Autodesk Inventor part; units mm, degrees
ref_plane "YZ Plane" through (0, 0, 0) normal (1, 0, 0) x (0, 1, 0)
ref_plane "XZ Plane" through (0, 0, 0) normal (0, 1, 0) x (-1, 0, 0)
ref_plane "XY Plane" through (0, 0, 0) normal (0, 0, 1) x (1, 0, 0)
sketch "Sketch1" plane through (0, 0, 0) normal (0, 0, 1) x (1, 0, 0)
  line L0 (-14.5, 25.1147) -> (14.5, 25.1147) construction
  line L1 (14.5, 25.1147) -> (29, 0) construction
  line L2 (29, 0) -> (14.5, -25.1147) construction
  line L3 (14.5, -25.1147) -> (-14.5, -25.1147) construction
  line L4 (-14.5, -25.1147) -> (-29, 0) construction
  line L5 (-29, 0) -> (-14.5, 25.1147) construction
  line L6 (-18.7639, 32.5) -> (18.7639, 32.5)
  line L7 (18.7639, 32.5) -> (37.5278, 0)
  line L8 (37.5278, 0) -> (18.7639, -32.5)
  line L9 (18.7639, -32.5) -> (-18.7639, -32.5)
  line L10 (-18.7639, -32.5) -> (-37.5278, 0)
  line L11 (-37.5278, 0) -> (-18.7639, 32.5)
  circle A0 centre (-14.5, 25.1147) radius 11 construction
  circle A1 centre (14.5, 25.1147) radius 11 construction
  circle A2 centre (29, 0) radius 11 construction
  circle A3 centre (14.5, -25.1147) radius 11 construction
  circle A4 centre (-14.5, -25.1147) radius 11 construction
  circle A5 centre (-29, 0) radius 11 construction
  circle A6 centre (-14.5, 25.1147) radius 4
  circle A7 centre (14.5, 25.1147) radius 4
  circle A8 centre (29, 0) radius 4
  circle A9 centre (14.5, -25.1147) radius 4
  circle A10 centre (-14.5, -25.1147) radius 4
  circle A11 centre (-29, 0) radius 4
  circle A12 centre (0, 0) radius 4
  circle A13 centre (0, 0) radius 40 construction
  circle A14 centre (0, 0) radius 37.5278 construction
  dimension "d17" = 75.0555
  dimension "d0" = 22
  dimension "d1" = 50.2295
  dimension "d2" = 8
  dimension "d3" = 65
  dimension "d4" = 8
  dimension "d13" = 80
extrude "Extrusion1" add sketch "Sketch1" along normal blind 5
fillet "Fillet1" radius 4 6 edges at (37.5278, 0, 2.5) (18.7639, -32.5, 2.5) (-18.7639, -32.5, 2.5) (-37.5278, 0, 2.5) (-18.7639, 32.5, 2.5) (18.7639, 32.5, 2.5)
sketch "Sketch2" plane through (0, 0, 5) normal (0, 0, 1) x (1, 0, 0)
  arc A0 (19.9186, 30.5) -> (16.4545, 32.5) centre (16.4545, 28.5) ccw
  line L0 (16.4545, 32.5) -> (-16.4545, 32.5)
  arc A1 (-16.4545, 32.5) -> (-19.9186, 30.5) centre (-16.4545, 28.5) ccw
  line L1 (-19.9186, 30.5) -> (-36.3731, 2)
  arc A2 (-36.3731, 2) -> (-36.3731, -2) centre (-32.909, 0) ccw
  line L2 (-36.3731, -2) -> (-19.9186, -30.5)
  arc A3 (-19.9186, -30.5) -> (-16.4545, -32.5) centre (-16.4545, -28.5) ccw
  line L3 (-16.4545, -32.5) -> (16.4545, -32.5)
  arc A4 (16.4545, -32.5) -> (19.9186, -30.5) centre (16.4545, -28.5) ccw
  line L4 (19.9186, -30.5) -> (36.3731, -2)
  arc A5 (36.3731, -2) -> (36.3731, 2) centre (32.909, 0) ccw
  line L5 (36.3731, 2) -> (19.9186, 30.5)
  circle A6 centre (0, 0) radius 4
  circle A7 centre (-29, 0) radius 4
  circle A8 centre (-14.5, -25.1147) radius 4
  circle A9 centre (14.5, -25.1147) radius 4
  circle A10 centre (29, 0) radius 4
  circle A11 centre (14.5, 25.1147) radius 4
  circle A12 centre (-14.5, 25.1147) radius 4
  circle A13 centre (0, 0) radius 4
  circle A14 centre (0, 0) radius 9
  dimension "d8" = 5
extrude "Extrusion2" add sketch "Sketch2" along normal blind 8 contours A7 | A8 | A9 | A10 | A11 | A12 | A14
sketch "Sketch3" plane through (0, 0, 0) normal (0, 0, -1) x (-1, 0, 0)
  circle A0 centre (0, 0) radius 4
  circle A1 centre (29, 0) radius 4
  circle A2 centre (14.5, -25.1147) radius 4
  circle A3 centre (-14.5, -25.1147) radius 4
  circle A4 centre (-29, 0) radius 4
  circle A5 centre (-14.5, 25.1147) radius 4
  circle A6 centre (14.5, 25.1147) radius 4
  arc A7 (-16.4545, 32.5) -> (-19.9186, 30.5) centre (-16.4545, 28.5) ccw
  line L0 (-19.9186, 30.5) -> (-36.3731, 2)
  arc A8 (-36.3731, 2) -> (-36.3731, -2) centre (-32.909, 0) ccw
  line L1 (-36.3731, -2) -> (-19.9186, -30.5)
  arc A9 (-19.9186, -30.5) -> (-16.4545, -32.5) centre (-16.4545, -28.5) ccw
  line L2 (-16.4545, -32.5) -> (16.4545, -32.5)
  arc A10 (16.4545, -32.5) -> (19.9186, -30.5) centre (16.4545, -28.5) ccw
  line L3 (19.9186, -30.5) -> (36.3731, -2)
  arc A11 (36.3731, -2) -> (36.3731, 2) centre (32.909, 0) ccw
  line L4 (36.3731, 2) -> (19.9186, 30.5)
  arc A12 (19.9186, 30.5) -> (16.4545, 32.5) centre (16.4545, 28.5) ccw
  line L5 (16.4545, 32.5) -> (-16.4545, 32.5)
extrude "Extrusion3" add sketch "Sketch3" against normal up to next contours A1 | A2 | A3 | A4 | A5 | A6
sketch "Sketch4" plane through (0, 0, 0) normal (0, 0, -1) x (-1, 0, 0)
  circle A0 centre (-14.5, 25.1147) radius 4 construction
  circle A1 centre (14.5, 25.1147) radius 4 construction
  circle A2 centre (29, 0) radius 4 construction
  circle A3 centre (14.5, -25.1147) radius 4 construction
  circle A4 centre (-14.5, -25.1147) radius 4 construction
  circle A5 centre (-29, 0) radius 4 construction
  circle A6 centre (-14.5, 25.1147) radius 1.35
  circle A7 centre (14.5, 25.1147) radius 1.35
  circle A8 centre (29, 0) radius 1.35
  circle A9 centre (14.5, -25.1147) radius 1.35
  circle A10 centre (-14.5, -25.1147) radius 1.35
  circle A11 centre (-29, 0) radius 1.35
  point P0 (0, 0)
  dimension "d14" = 2.7
extrude "Extrusion4" cut sketch "Sketch4" against normal through all
properties part number "rotor 2"
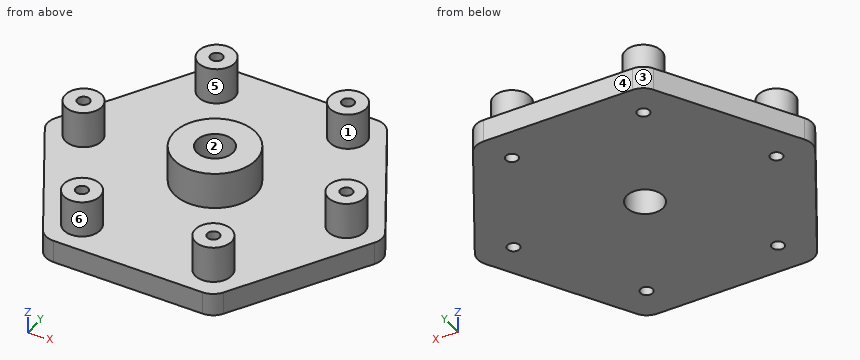
Check sheet for the modelled part. Datum: model origin and axes. Units: mm. Face numbers are marked on the shaded views. A direction names the side the tool comes from. Coordinates: 2 decimals unless noted, no trailing zeros. Loops run counter-clockwise (first coordinate to the right, second up) from the corner with the lowest first, then second, coordinate; pieces in that order, holes last.
1) Sectioned sample at A-A (y = 0). Record the boundary of the cut face in (x, z).
2) Gauge pin test, flat ends, axial feed: pin 1 (3 mm diameter, centred on x = -18, y = 26, fed in from -Z); pin 2 (5 mm diameter, centred on x = -29, z = 4.5, fed in from +Y); pin 3 (3 mm diameter, centred on x = -19.5, y = 4.5, fed in from +Z); pin 4 (1.5 mm diameter, centred on y = 25.5, z = 9.5, fed in from +X). Record the tip position at first contact, or that the pin passes through.
3) Sectioned sample at C-C (z = 11.25). Count the separate pieces of the cut face and the enclosed holes in it, and give its area (3 significant figures).
4) Material ranges on probe 1 along Y at (x, z) = (14.5, 8.25); probe 2 along Y at (x, z) = (-14.5, 3); probe 3 along X at (y, z) = (0.5, 8), recorded low to high.
5) Sectioned sample at B-B (x = 14.5). Record the boundary of the cut face in (y, z).
6) Access from +Z, -Z, +X, -X, +Y, -Y to the whole of each face (thin tool, end or side, straight path). Record for the marked faces 1 and 2.
7) Sectioned sample at D-D (x = 0). Record the boundary of the cut face in (y, z), and give its area (3 significant figures).
8) Release check for a two-part mould opening along X. For the marked faces 3, 4, 5 and 6 record: released by +X, released by -X, zero draft, split by the parting line, or undercut.
Check sheet entries:
1. outline: (-36.91, 0) - (-30.35, 0) - (-30.35, 13) - (-33, 13) - (-33, 5) - (-36.91, 5) - close; (-27.65, 0) - (-4, 0) - (-4, 13) - (-9, 13) - (-9, 5) - (-25, 5) - (-25, 13) - (-27.65, 13) - close; (4, 0) - (27.65, 0) - (27.65, 13) - (25, 13) - (25, 5) - (9, 5) - (9, 13) - (4, 13) - close; (30.35, 0) - (36.91, 0) - (36.91, 5) - (33, 5) - (33, 13) - (30.35, 13) - close
2. pin 1: stops at z = 0
2. pin 2: stops at y = 19.1
2. pin 3: stops at z = 5
2. pin 4: stops at x = 18.5
3. separate pieces: 7
3. enclosed holes: 7
3. area: 471 mm2
4. probe 1: y = -29.11 to -26.46, -23.76 to -21.11, 21.11 to 23.76, 26.46 to 29.11
4. probe 2: y = -32.5 to -26.46, -23.76 to 23.76, 26.46 to 32.5
4. probe 3: x = -32.97 to -30.25, -27.75 to -25.03, -8.99 to -3.97, 3.97 to 8.99, 25.03 to 27.75, 30.25 to 32.97
5. outline: (-32.5, 0) - (-26.46, 0) - (-26.46, 13) - (-29.11, 13) - (-29.11, 5) - (-32.5, 5) - close; (-23.76, 0) - (23.76, 0) - (23.76, 13) - (21.11, 13) - (21.11, 5) - (-21.11, 5) - (-21.11, 13) - (-23.76, 13) - close; (26.46, 0) - (32.5, 0) - (32.5, 5) - (29.11, 5) - (29.11, 13) - (26.46, 13) - close
6. face 1: +Z
6. face 2: +Z, -Z
7. outline: (-32.5, 0) - (-4, 0) - (-4, 13) - (-9, 13) - (-9, 5) - (-32.5, 5) - close; (4, 0) - (32.5, 0) - (32.5, 5) - (9, 5) - (9, 13) - (4, 13) - close
7. area: 365 mm2
8. face 3: released by -X
8. face 4: zero draft
8. face 5: undercut
8. face 6: undercut
